Source: three-view drawing plus pictorial views. Frame: mm from the lowest corner of the part. Give positions to 0.01 mm unless a question says otherwise; leave off trailing zeros. Write each loop counter-clockwise with the first axis right and the second up, starting at its lowest first coordinate (ties: lowest second). Pieces come first, ordered by that corner, then holes. Notation, with made-up numbers: (52, 52) -> (79, 52) arc R26 ccw to (79, 87) -> close; hole circle Ø4 at (-13, 8.5). An arc over 180 degrees is marked (long way). Answer in a Markdown table with one row per item. Add a question column.
Item 1: Draft query along Z for the marked faces 1, 2 and 3. Return one class per face: +Z half, -Z half, draft (parallel to the pull), parting line (faces both ways), or undercut.
Item 2: Section query C-C on x = 6. Output: boundary loops of the cut face in (y, z).
Item 3: Section query B-B on z = 26. Output: boundary loops of the cut face in (x, y), plus the area to 3 significant figures.
Item 4: Section query A-A on x = 16. Output: boundary loops of the cut face in (y, z), plus the area to 3 significant figures.
Item 5: Section query D-D on y = 1.5. Output: boundary loops of the cut face in (x, z).
Item 6: Material intervals for probe 1 along Z at (x, y) = (16, 2.7); probe 2 along Y at (x, z) = (16, 1); probe 3 along X at (y, z) = (6, 26), sorted ascending. Write a range as from..to.
Item 7: First-contact query: P1, Ø2, axis at x = 28.5, y = 9.5, coming from the +Z side; P2, Ø10, axis at x = 19.5, z = 8.5, coming from the +Y side; P3, Ø2, axis at x = 21, y = 4.5, coming from the -Z side. Flat tips, straight axial feed; report the tip coordinate or a pass-through.
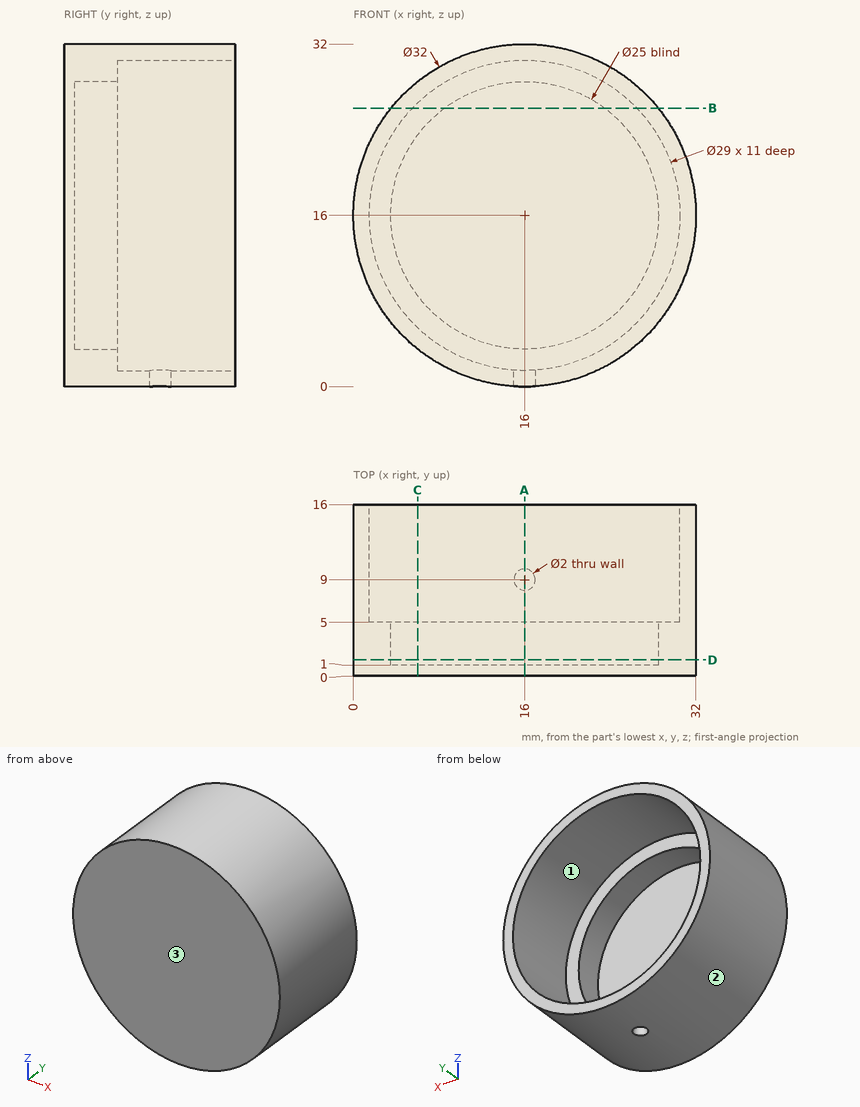
Findings below:
| question | item | result |
|---|---|---|
| 1 | face 1 | undercut |
| 1 | face 2 | parting line |
| 1 | face 3 | draft |
| 2 | outline | (0, 3.51) -> (16, 3.51) -> (16, 5.5) -> (5, 5.5) -> (5, 8.5) -> (1, 8.5) -> (1, 23.5) -> (5, 23.5) -> (5, 26.5) -> (16, 26.5) -> (16, 28.49) -> (0, 28.49) -> close |
| 3 | outline | (3.51, 0) -> (28.49, 0) -> (28.49, 16) -> (26.5, 16) -> (26.5, 5) -> (23.5, 5) -> (23.5, 1) -> (8.5, 1) -> (8.5, 5) -> (5.5, 5) -> (5.5, 16) -> (3.51, 16) -> close |
| 3 | area | 109 mm^2 |
| 4 | outline | (0, 0) -> (8, 0) -> (8, 1.5) -> (5, 1.5) -> (5, 3.5) -> (1, 3.5) -> (1, 28.5) -> (5, 28.5) -> (5, 30.5) -> (16, 30.5) -> (16, 32) -> (0, 32) -> close; (10, 0) -> (16, 0) -> (16, 1.5) -> (10, 1.5) -> close |
| 4 | area | 90.0 mm^2 |
| 5 | outline | circle Ø32 at (16, 16); hole circle Ø25 at (16, 16) |
| 6 | probe 1 | z = 0..3.5, 28.5..32 |
| 6 | probe 2 | y = 0..8, 10..16 |
| 6 | probe 3 | x = 3.51..5.5, 26.5..28.49 |
| 7 | P1 | stops at z = 27.12 |
| 7 | P2 | stops at y = 5 |
| 7 | P3 | stops at z = 0.51 |
